Can you work these out from the model? Positions are in its coordinate system, mm. A direction names the side the tool comes from. Give positions to 0.01 mm unless a question says otherwise; leave off trailing zeros. Write each loop counter-clockwise with the first axis right and the second up, starting at its lowest first coordinate (ties: lowest second). Pieces come first, ordered by that corner, then holes.
Autodesk Inventor part; units mm, degrees
ref_plane "YZ Plane" through (0, 0, 0) normal (1, 0, 0) x (0, 1, 0)
ref_plane "XZ Plane" through (0, 0, 0) normal (0, 1, 0) x (-1, 0, 0)
ref_plane "XY Plane" through (0, 0, 0) normal (0, 0, 1) x (1, 0, 0)
sketch "Sketch1" plane through (0, 0, 0) normal (0, 0, 1) x (1, 0, 0)
  line L0 (-73.025, 0) -> (-73.025, 25.4)
  line L1 (-73.025, 25.4) -> (73.025, 25.4)
  line L2 (73.025, 25.4) -> (73.025, 0)
  line L3 (73.025, 0) -> (35.4919, 0)
  line L4 (-73.025, 0) -> (-35.4919, 0)
  arc A0 (35.4919, 0) -> (-35.4919, 0) centre (0, -38.1) ccw
  point P0 (0, 0)
  dimension "d1" = 104.14
  dimension "d2" = 38.1
  dimension "d3" = 146.05
  dimension "d4" = 25.4
extrude "Extrusion1" add sketch "Sketch1" along normal blind 25.4
sketch "Sketch2" plane through (-73.025, 25.4, 0) normal (0, 1, 0) x (1, 0, 0)
  line L0 (0, 0) -> (146.05, 0) construction
  line L1 (0, 0) -> (0, -25.4) construction
  line L2 (146.05, -25.4) -> (0, -25.4) construction
  line L3 (146.05, 0) -> (146.05, -25.4) construction
  circle A0 centre (12.7, -12.7) radius 3.4925
  circle A1 centre (133.35, -12.7) radius 3.4925
  point P0 (73.025, 0)
  dimension "d7" = 6.985
  dimension "d8" = 6.985
  dimension "d9" = 12.7
  dimension "d10" = 12.7
extrude "Extrusion2" cut sketch "Sketch2" against normal through all
fillet "Fillet1" radius 3.175 6 edges at (73.025, 25.4, 12.7) (-73.025, 25.4, 12.7) (-73.025, 0, 12.7) (-35.4919, 0, 12.7) (35.4919, 0, 12.7) (73.025, 0, 12.7)
sketch "Sketch3" plane through (-69.85, 25.4, 0) normal (0, 1, 0) x (1, 0, 0)
  line L0 (0, -25.4) -> (0, 0) construction
  line L1 (139.7, -25.4) -> (0, -25.4) construction
  line L2 (139.7, 0) -> (139.7, -25.4) construction
  line L3 (0, 0) -> (139.7, 0) construction
  circle A0 centre (9.525, -12.7) radius 3.4925 construction
  circle A1 centre (130.175, -12.7) radius 3.4925 construction
  circle A2 centre (9.525, -12.7) radius 3.4925
  circle A3 centre (9.525, -12.7) radius 6.35
  circle A4 centre (130.175, -12.7) radius 6.35
  point P0 (69.85, 0)
  dimension "d14" = 12.7
  dimension "d15" = 12.7
extrude "Extrusion3" cut sketch "Sketch3" against normal blind 7.62
properties part number "Top" material "ABS Plastic"
(1) For faces 5 (the face through (72.12, 24.445, 12.878)), 6 (the face through (66.19, 21.64, 15.13)), which set-ups out of +Z, -Z, +X, -X, +Y, -Y let a thin tool reach every point of the face, with its end or its side?
Returned:
face 5: +Z, -Z, +X, +Y
face 6: +Y
(2) If we mould it in two halves opening along Z, with no side actions, what happens to faces 1 (the face through (-63.814, 9.014, 12.546)), 2 (the face through (-1, 16, 25.4)), 3 (the face through (-72.07, 24.495, 12.878)), 4 (the face through (63.656, 9.014, 11.651))? For each: +Z half, -Z half, draft (parallel to the pull), parting line (faces both ways), or undercut.
Returned:
face 1: undercut
face 2: +Z half
face 3: draft
face 4: undercut
(3) Will these pins go through, and if not, where does the flat tip stop? P1, Ø6.5, axis at x = -58.5, z = 11, coming from the +Y side; P2, Ø6, axis at x = -32.5, z = 11.5, coming from the -Y side; P3, Ø6.5, axis at x = -60.325, z = 12.7, coming from the -Y side.
Returned:
P1: stops at y = 17.78
P2: stops at y = 0.24
P3: passes through
(4) Imagine slicing it at D-D, the plane y = 20.5. Write out the boundary of the cut face in (x, z) (3 decimals).
Returned:
outline: (-73.025, 0) - (73.025, 0) - (73.025, 25.4) - (-73.025, 25.4) - close; hole circle Ø12.7 at (-60.325, 12.7); hole circle Ø12.7 at (60.325, 12.7)
(5) Imagine slicing it at B-B, the plane y = 11.5. Write out the boundary of the cut face in (x, z) (1 decimal), plus the area to 3 significant figures.
Returned:
outline: (-73, 0) - (-15.8, 0) - (-15.8, 25.4) - (-73, 25.4) - close; (15.8, 0) - (73, 0) - (73, 25.4) - (15.8, 25.4) - close; hole circle Ø7 at (-60.3, 12.7); hole circle Ø7 at (60.3, 12.7)
area: 2,830 mm2
(6) Imagine slicing it at A-A, the plane z = 12.7. Give the number of separate pieces and of enclosed holes in the cut face, plus the area to 3 significant figures.
Returned:
separate pieces: 3
enclosed holes: 0
area: 2,580 mm2
(7) If I drill on L1, parallel to X at y = 24.25, z = 11.5; L2, parallel to Y at x = 0, z = 7.5; L3, parallel to X at y = 22.5, z = 11, over which ranges is the centre line in solid material (lowest first)?
Returned:
L1: x = -72.3 to -66.56, -54.09 to 54.09, 66.56 to 72.3
L2: y = 13.97 to 25.4
L3: x = -73.01 to -66.44, -54.21 to 54.21, 66.44 to 73.01
(8) Imagine slicing it at C-C, the plane z = 22. Write out the boundary of the cut face in (x, y) (3 decimals), plus the area to 3 significant figures.
Returned:
outline: (-73.025, 3.175) arc R3.175 ccw to (-69.85, 0) - (-36.72, 0) arc R3.175 ccw to (-34.61, 0.803) arc R52.07 cw to (34.61, 0.803) arc R3.175 ccw to (36.72, 0) - (69.85, 0) arc R3.175 ccw to (73.025, 3.175) - (73.025, 22.225) arc R3.175 ccw to (69.85, 25.4) - (-69.85, 25.4) arc R3.175 ccw to (-73.025, 22.225) - close
area: 3,020 mm2
